Autodesk Inventor part; units mm, degrees
ref_plane "YZ Plane" through (0, 0, 0) normal (1, 0, 0) x (0, 1, 0)
ref_plane "XZ Plane" through (0, 0, 0) normal (0, 1, 0) x (-1, 0, 0)
ref_plane "XY Plane" through (0, 0, 0) normal (0, 0, 1) x (1, 0, 0)
sketch "Base Profile" plane through (0, 0, 0) normal (0, 1, 0) x (-1, 0, 0)
  line L0 (0, 0) -> (15, 0)
  line L1 (15, 0) -> (15, -15)
  line L2 (15, -15) -> (0, -15)
  line L3 (0, -15) -> (0, 0)
  line L4 (15, 0) -> (27, 0)
  line L5 (27, 0) -> (27, -15)
  line L6 (27, -15) -> (15, -15)
  dimension "d413" = 15
  dimension "d414" = 15
  dimension "d417" = 12
extrude "Stock" add sketch "Base Profile" against normal blind 33
extrude "Extrusion Post" add sketch "Base Profile" along normal blind 15 contours L0 L1 L2 L3
sketch "Sketch39" plane through (0, 15, 0) normal (0, 1, 0) x (1, 0, 0)
  line L0 (0, 15) -> (-15, 15)
  line L1 (-15, 15) -> (-15, 0)
  line L2 (-15, 0) -> (0, 0)
  line L3 (0, 0) -> (0, 15)
  circle A0 centre (-7.5, 7.5) radius 3.175
  point P0 (0, 7.5)
  point P1 (-7.5, 0)
  dimension "d418" = 6.35
hole "Hole27" at (-7.5, 15, -7.5) direction (0, -1, 0) diameter 3.2004 end through all counterbore diameter 6.5024 counterbore depth 2.9972
equation "\"d168\" = extrusionOffset"
equation "\"extrusionWidth\" = 15"
equation "\"idlerLength\" = 12"
equation "\"bearingOffsetFromBottom\" = 7.5"
equation "\"extrusionOffset\" = 33"
equation "\"bearingStackHeight\" = 9"
equation "\"bearingClearance\" = 13"
equation "\"pinSupportLength\" = 2"
properties part number "A Idler" material "Aluminum 6061"
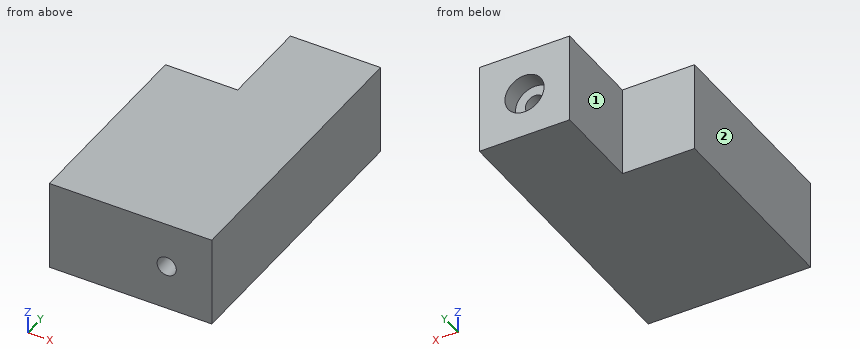
Read the model definition and answer for the solid it produces. Units are mm, in the model's axes. Face numbers are marked on the shaded views. A direction names the side the tool comes from. Round coordinates to 2 decimals unless told otherwise and drop trailing zeros. Write each loop counter-clockwise with the first axis right and the second up, starting at its lowest first coordinate (ties: lowest second). Pieces come first, ordered by that corner, then holes.
Q1. Find section B-B on x = -7.5. Determine the outline of the cut face in (y, z), and give its area (3 significant figures).
Values:
outline: (-33, -15) - (15, -15) - (15, -10.75) - (12, -10.75) - (12, -9.1) - (-33, -9.1) - close; (-33, -5.9) - (12, -5.9) - (12, -4.25) - (15, -4.25) - (15, 0) - (-33, 0) - close
area: 556 mm2
Q2. Flat-ended cylindrical pins translate along their axes: P1, Ø2, axis at x = -21, z = -3, coming from the +Y side; P2, Ø4.5, axis at y = 10.5, z = -7.5, coming from the -X side; P3, Ø2, axis at x = -7.5, z = -6, coming from the +Y side. Find the tip coordinate at first contact, or state that the pin passes through.
Values:
P1: stops at y = 0
P2: stops at x = -15
P3: stops at y = 12
Q3. Find section A-A on z = -7.5. Determine the outline of the cut face in (x, y), and give its area (3 significant figures).
Values:
outline: (-27, -33) - (-9.1, -33) - (-9.1, 12) - (-10.75, 12) - (-10.75, 15) - (-15, 15) - (-15, 0) - (-27, 0) - close; (-5.9, -33) - (0, -33) - (0, 15) - (-4.25, 15) - (-4.25, 12) - (-5.9, 12) - close
area: 952 mm2
Q4. Straight lines are drawn through the part: line 1 (Z direction, x = -7.5, y = 13.4); line 2 (X direction, y = -6, z = -7.5). For each, find the intervals that lie inside material, in ascending order.
Values:
line 1: z = -15 to -10.75, -4.25 to 0
line 2: x = -27 to -9.1, -5.9 to 0
Q5. Find section C-C on y = -23. Determine the outline of the cut face in (x, z), and give its area (3 significant figures).
Values:
outline: (-27, -15) - (0, -15) - (0, 0) - (-27, 0) - close; hole circle Ø3.2 at (-7.5, -7.5)
area: 397 mm2
Q6. A tool of negligible diameter and unlimited length cuts with its end or side. For the marked faces 1 and 2, from which of +Z, -Z, +X, -X, +Y, -Y can it reach the whole face along a straight path? Write none if from no direction.
Values:
face 1: +Z, -Z, -X, +Y
face 2: +Z, -Z, -X, +Y, -Y
Q7. Find section D-D on x = -17. Determine the outline of the cut face in (y, z).
Values:
outline: (-33, -15) - (0, -15) - (0, 0) - (-33, 0) - close
